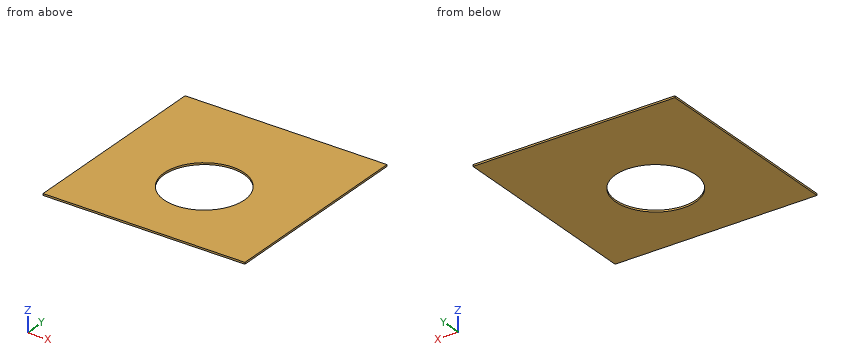
Autodesk Inventor part; units mm, degrees
ref_plane "YZ Plane" through (0, 0, 0) normal (1, 0, 0) x (0, 1, 0)
ref_plane "XZ Plane" through (0, 0, 0) normal (0, 1, 0) x (-1, 0, 0)
ref_plane "XY Plane" through (0, 0, 0) normal (0, 0, 1) x (1, 0, 0)
sketch "Sketch1" plane through (0, 0, 0) normal (0, 0, 1) x (1, 0, 0)
  line L0 (-3.4369, 182.883) -> (106.5631, 182.883)
  line L1 (106.5631, 182.883) -> (106.5631, 42.883)
  line L2 (106.5631, 42.883) -> (-3.4369, 42.883)
  line L3 (-3.4369, 42.883) -> (-3.4369, 182.883)
  circle A0 centre (51.5631, 76.8468) radius 15.875
  line L4 (-3.4369, 122.883) -> (106.5631, 122.883)
  line L5 (91.5631, 122.883) -> (91.5631, 42.883)
  line L6 (11.5631, 122.883) -> (11.5631, 42.883)
  point P0 (0, 0)
  point P1 (51.5631, 42.883)
  dimension "d0" = 140
  dimension "d1" = 110
  dimension "d2" = 31.75
  dimension "d5" = 80
  dimension "d6" = 15
  dimension "d7" = 15
extrude "Extrusion1" add sketch "Sketch1" against normal blind 0.7 contours L4 L5 L2 L6
equation "\"d7\" = d6"
properties part number "cage_wall"
Model file for the job. Use its own axes, mm. Round coordinates to 2 decimals unless told otherwise and drop trailing zeros. Loops run counter-clockwise (first coordinate to the right, second up) from the corner with the lowest first, then second, coordinate; pieces in that order, holes last. Notation, with made-up numbers: (65.25, -33) -> (80.25, -33) arc R33 cw to (80.25, 1) -> close; hole circle Ø1 at (56.25, -14). An arc over 180 degrees is marked (long way). Answer as CSV lines item,"result". Start each with the question number.
1) Slice it at A-A (x = 40.5). List the corners of the cut face in (y, z), plus the area to 3 significant figures.
2) Slice it at B-B (y = 72.5). List the corners of the cut face in (x, z), plus the area to 3 significant figures.
3) Slice it at C-C (z = -0.4). List the corners of the cut face in (x, y) (3 decimals).
4) Pin check, flat tip, straight feed: P1, Ø19, axis at x = 51.56, y = 76.85, coming from the -Z side (3 decimals). Stop position of the tip, or through.
5) Probe line 1 along Y through (x, z) = (42, -0.5); line 2 along Y through (x, z) = (43.5, -0.25); line 3 along X through (y, z) = (91, -0.1). List the from-to ranges inside material, lowest first.
Filled in:
1,outline,"(42.88, -0.7) -> (65.46, -0.7) -> (65.46, 0) -> (42.88, 0) -> close; (88.23, -0.7) -> (122.88, -0.7) -> (122.88, 0) -> (88.23, 0) -> close"
1,area,"40.1 mm2"
2,outline,"(11.56, -0.7) -> (36.29, -0.7) -> (36.29, 0) -> (11.56, 0) -> close; (66.83, -0.7) -> (91.56, -0.7) -> (91.56, 0) -> (66.83, 0) -> close"
2,area,"34.6 mm2"
3,outline,"(11.563, 42.883) -> (91.563, 42.883) -> (91.563, 122.883) -> (11.563, 122.883) -> close; hole circle Ø31.75 at (51.563, 76.847)"
4,P1,"passes through"
5,line 1,"y = 42.88 to 64.18, 89.52 to 122.88"
5,line 2,"y = 42.88 to 63.17, 90.52 to 122.88"
5,line 3,"x = 11.56 to 44.37, 58.75 to 91.56"
